Here's how the part is built. I have some questions about the finished solid (model axes, mm). A direction names the side the tool comes from. Coordinates: 2 decimals unless noted, no trailing zeros. Write each loop counter-clockwise with the first axis right and the second up, starting at its lowest first coordinate (ties: lowest second). Pieces come first, ordered by that corner, then holes.
(1) For pin 1 Ø1 at (x, y) = (15.5, 1) entering from +Z; pin 2 Ø6.5 at (y, z) = (5, -4) entering from +X; pin 3 Ø3 at (x, y) = (17.5, 3.5) entering from -Z; pin 4 Ø2.5 at (x, z) = (23.5, -6.125) entering from +Y, each with a flat end and sliding along its axis, tell me the tip position at first contact or that it passes through.
(2) Please list where these lines run through material, in increasing order: probe 1 along Z at (x, y) = (23.5, 6.2) (3 decimals); probe 2 along Y at (x, z) = (13, -9) (3 decimals); probe 3 along X at (y, z) = (4, -11).
(3) Which directions (+Z, -Z, +X, -X, +Y, -Y) give clear straight access to the entire face, cutting with the end or side of a thin tool? Please do faces 1 (the flat face through (0, 8, 3.825)), 2 (the flat face through (20, -6, -2.975)), 3 (the cylindrical face through (12.215, 8.049, 3.524)).
(4) Imagine slicing it at A-A, the plane x = 23.5. List the corners of the cut face in (y, z) for me (3 decimals).
(5) Imagine slicing it at B-B, the plane z = -1.75. List the corners of the cut face in (x, y) for me.
(6) Imagine slicing it at C-C, the plane x = 5. List the corners of the cut face in (y, z) for me (3 decimals), plus the area to 3 significant figures.
```python
from build123d import *

# Parameters (mm, degrees)
F1_DEPTH = 12.5
F2_W     = 1.45
F2_H     = 6.3
F2_R     = 2.3
F3_DEPTH = 28.5
F4_R     = 1.5
F5_DEPTH = 12.5
F6_SIZE  = 0.5
F7_R     = 2.3
F8_DEPTH = 4
F9_R     = 2
F10_R    = 1


with BuildPart() as f1:
    # F0 (on Right) → F1 (new body, symmetric)
    with BuildSketch(Plane.YZ):
        with BuildLine():
            Line((-9, -12.25), (9, -12.25))
            ThreePointArc((9, -12.25), (11.12132, -11.37132), (12, -9.25))
            Line((12, -9.25), (12, 0.825))
            ThreePointArc((12, 0.825), (11.12132, 2.94632), (9, 3.825))
            Line((9, 3.825), (6.125, 3.825))
            Line((6.125, 3.825), (6.125, 6.125))
            ThreePointArc((6.125, 6.125), (0, 12.25), (-6.125, 6.125))
            Line((-6.125, 6.125), (-6.125, 3.825))
            Line((-6.125, 3.825), (-9, 3.825))
            ThreePointArc((-9, 3.825), (-11.12132, 2.94632), (-12, 0.825))
            Line((-12, 0.825), (-12, -9.25))
            ThreePointArc((-12, -9.25), (-11.12132, -11.37132), (-9, -12.25))
        make_face()
    extrude(amount=F1_DEPTH, both=True)

    # F2 (on Right) → F3 (join)
    with BuildSketch(Plane.YZ):
        with Locations((-6.35, -6.125)):
            Rectangle(F2_W, F2_H)
        with Locations((6.35, -6.125)):
            Rectangle(F2_W, F2_H)
        with Locations((0, 6.125)):
            Circle(F2_R)
    extrude(amount=F3_DEPTH)

    # F4 (on Front) → F5 (cut, symmetric)
    with BuildSketch(Plane.XZ):
        with Locations((23.5, -6.125)):
            Circle(F4_R)
    extrude(amount=F5_DEPTH, both=True, mode=Mode.SUBTRACT)

    # F6
    f6_edges = [f1.edges().sort_by_distance(p)[0] for p in [
        (28.5, -7.075, -6.125),
        (28.5, -6.35, -9.275),
        (28.5, -5.625, -6.125),
        (28.5, -6.35, -2.975),
        (28.5, 5.625, -6.125),
        (28.5, 6.35, -9.275),
        (28.5, 7.075, -6.125),
        (28.5, 6.35, -2.975),
    ]]
    chamfer(f6_edges, length=F6_SIZE)

    # F7 (on face) → F8 (join)
    with BuildSketch(Plane.YZ.offset(28.5)):
        with Locations((0, 6.125)):
            Circle(F7_R)
    extrude(amount=F8_DEPTH)

    # F9
    f9_edges = [f1.edges().sort_by_distance(p)[0] for p in [
        (32.5, -2.3, 6.125),
    ]]
    fillet(f9_edges, radius=F9_R)

    # F10
    f10_edges = [f1.edges().sort_by_distance(p)[0] for p in [
        (12.5, 0, 12.25),
        (12.5, 7.5625, 3.825),
        (-12.5, 11.12132, -11.37132),
        (-12.5, 0, 12.25),
        (0, -6.125, 3.825),
        (0, 6.125, 3.825),
    ]]
    fillet(f10_edges, radius=F10_R)


solid = f1.part
```
Recorded:
1. pin 1: stops at z = 8.37
1. pin 2: stops at x = 28.5
1. pin 3: stops at z = 4.99
1. pin 4: passes through
2. probe 1: z = -9.275 to -7.625, -4.625 to -2.975
2. probe 2: y = -7.075 to -5.625, 5.625 to 7.075
2. probe 3: x = -12.5 to 12.5
3. face 1: +Z, +X, -X, +Y
3. face 2: +Z, +X, +Y, -Y
3. face 3: +Z, +X, +Y
4. outline: (-7.075, -9.275) - (-5.625, -9.275) - (-5.625, -7.625) - (-7.075, -7.625) - close; (-7.075, -4.625) - (-5.625, -4.625) - (-5.625, -2.975) - (-7.075, -2.975) - close; circle Ø4.6 at (0, 6.125); (5.625, -9.275) - (7.075, -9.275) - (7.075, -7.625) - (5.625, -7.625) - close; (5.625, -4.625) - (7.075, -4.625) - (7.075, -2.975) - (5.625, -2.975) - close
5. outline: (-12.5, -11) arc R1 ccw to (-11.5, -12) - (11.5, -12) arc R1 ccw to (12.5, -11) - (12.5, 11) arc R1 ccw to (11.5, 12) - (-11.5, 12) arc R1 ccw to (-12.5, 11) - close
6. outline: (-12, -9.25) arc R3 ccw to (-9, -12.25) - (9, -12.25) arc R3 ccw to (12, -9.25) - (12, 0.825) arc R3 ccw to (9, 3.825) - (7.125, 3.825) arc R1 cw to (6.125, 4.825) - (6.125, 6.125) arc R6.125 ccw to (-6.125, 6.125) - (-6.125, 4.825) arc R1 cw to (-7.125, 3.825) - (-9, 3.825) arc R3 ccw to (-12, 0.825) - close
6. area: 466 mm2
